The listing builds one solid part. Answer for the finished solid, in the listing's coordinates (mm). Coordinates: 2 decimals unless noted, no trailing zeros. Order: outer loops, then holes, each group sorted by start corner. A loop starts at its lowest first (then second) coordinate and runs counter-clockwise, first axis right, second up. Notation, with made-up numbers: (-24, -28) -> (23, -28) arc R16 ccw to (23, -23) -> close; hole circle Ø3 at (42, -14.75). An arc over 180 degrees is marked (long way). Answer in a Markdown table with one row per item.
```python
from build123d import *

# Parameters (mm, degrees)
SKETCH1_W               = 150
SKETCH1_H               = 150
BOSS_EXTRUDE1_DEPTH     = 7.5
SKETCH2_R               = 3.075
CUT_EXTRUDE2_DEPTH      = 32
SKETCH5_R               = 10
CUT_EXTRUDE5_DEPTH      = 22
SKETCH6_R               = 3.25
CUT_EXTRUDE6_DEPTH      = 22
MIRROR2_COPY_1_SKETCH_R = 3.25
MIRROR2_COPY_1_DEPTH    = 22


with BuildPart() as part:
    # Sketch1 → Boss-Extrude1 (new, symmetric)
    with BuildSketch(Plane.XY):
        Rectangle(SKETCH1_W, SKETCH1_H)
    extrude(amount=BOSS_EXTRUDE1_DEPTH, both=True)

    # Sketch2 → Cut-Extrude2 (cut)
    with BuildSketch(Plane(origin=(0, 0, -7.5), x_dir=(-1, 0, 0), z_dir=(0, 0, -1))):
        with Locations((52.5, 61)):
            Circle(SKETCH2_R)
    extrude(amount=-CUT_EXTRUDE2_DEPTH, mode=Mode.SUBTRACT)

    # Sketch5 → Cut-Extrude5 (cut)
    with BuildSketch(Plane.XY.offset(7.5)):
        with Locations((-48.369109736, 0)):
            Circle(SKETCH5_R)
    extrude(amount=-CUT_EXTRUDE5_DEPTH, mode=Mode.SUBTRACT)

    # Sketch6 → Cut-Extrude6 (cut)
    with BuildSketch(Plane(origin=(0, 0, -7.5), x_dir=(-1, 0, 0), z_dir=(0, 0, -1))):
        with Locations((69, 69)):
            Circle(SKETCH6_R)
    cut_extrude6 = extrude(amount=-CUT_EXTRUDE6_DEPTH, mode=Mode.SUBTRACT)

    # Mirror1: Cut-Extrude6 across plane
    add(cut_extrude6.mirror(Plane.ZX), mode=Mode.SUBTRACT)

    # Mirror2: Cut-Extrude6 across plane
    add(cut_extrude6.mirror(Plane(origin=(0, 0, 0), x_dir=(0, 0, 1), z_dir=(1, 0, 0))), mode=Mode.SUBTRACT)

    # Mirror2 copy 1 sketch → Mirror2 copy 1 (cut)
    with BuildSketch(Plane(origin=(0, 0, -7.5), x_dir=(1, 0, 0), z_dir=(0, 0, -1))):
        with Locations((69, 69)):
            Circle(MIRROR2_COPY_1_SKETCH_R)
    extrude(amount=-MIRROR2_COPY_1_DEPTH, mode=Mode.SUBTRACT)


solid = part.part
```
(1) For a pull along X with two mould halves and no side action, classify faces 1 (the flat face through (-75, -1, 0)), 2 (the flat face through (-1, 75, 0)), 3 (the cylindrical face through (-55.34, 59.82, -0.11)), 4 (the cylindrical face through (66.421, -67.022, -0.105)) as released by +X, released by -X, zero draft, split by the parting line, or undercut.
Check values:
| item | result |
|---|---|
| face 1 | released by -X |
| face 2 | zero draft |
| face 3 | undercut |
| face 4 | undercut |
(2) A cutting plane is placed at A-A, the plane x = 69. Determine the outline of the cut face in (y, z), then the cut area to 4 significant figures.
Check values:
| item | result |
|---|---|
| outline | (-75, -7.5) -> (-72.25, -7.5) -> (-72.25, 7.5) -> (-75, 7.5) -> close; (-65.75, -7.5) -> (65.75, -7.5) -> (65.75, 7.5) -> (-65.75, 7.5) -> close; (72.25, -7.5) -> (75, -7.5) -> (75, 7.5) -> (72.25, 7.5) -> close |
| area | 2,055 mm² |
(3) A flat-ended cylindrical pin translates along its axis: pin 1 (8.5 mm diameter, centred on x = 69, y = -69, fed in from -Z). Find the tip coordinate at first contact, or state that the pin passes through.
Check values:
| item | result |
|---|---|
| pin 1 | z = -7.5 |
(4) A cutting plane is placed at C-C, the plane y = 61. Determine the outline of the cut face in (x, z) (3 decimals), then the cut area to 3 significant figures.
Check values:
| item | result |
|---|---|
| outline | (-75, -7.5) -> (-55.575, -7.5) -> (-55.575, 7.5) -> (-75, 7.5) -> close; (-49.425, -7.5) -> (75, -7.5) -> (75, 7.5) -> (-49.425, 7.5) -> close |
| area | 2,160 mm² |
(5) A cutting plane is placed at D-D, the plane z = -5. Determine the outline of the cut face in (x, y) (3 decimals), then the cut area to 3 significant figures.
Check values:
| item | result |
|---|---|
| outline | (-75, -75) -> (75, -75) -> (75, 75) -> (-75, 75) -> close; hole circle Ø6.5 at (-69, -69); hole circle Ø6.5 at (-69, 69); hole circle Ø20 at (-48.369, 0); hole circle Ø6.15 at (-52.5, 61); hole circle Ø6.5 at (69, -69); hole circle Ø6.5 at (69, 69) |
| area | 22,000 mm² |
(6) Find the intervals of material crossed by line 1 along Y through (x, z) = (69, 0); line 2 along Y through (x, z) = (-52.5, 1.5) (3 decimals); line 3 along X through (y, z) = (-68, 1.75), in increasing order. Write a range as from..to.
Check values:
| item | result |
|---|---|
| line 1 | -75..-72.25, -65.75..65.75, 72.25..75 |
| line 2 | -75..-9.107, 9.107..57.925, 64.075..75 |
| line 3 | -75..-72.09, -65.91..65.91, 72.09..75 |
